Can you work these out from the drawing? Everything is in mm from the part's minimum corner. Give positions to 0.01 mm unless a question says otherwise; leave off trailing zeros. Order: outer loops, then holes, each group sorted by start corner. A loop starts at its lowest first (then second) coordinate and runs counter-clockwise, first axis right, second up. Notation, with made-up numbers: (63, -33.5) -> (87, -33.5) arc R31 ccw to (87, -5.5) -> close; hole circle Ø10 at (-26, -10.5). An arc over 180 degrees is marked (long way). One line per item, written item: value.
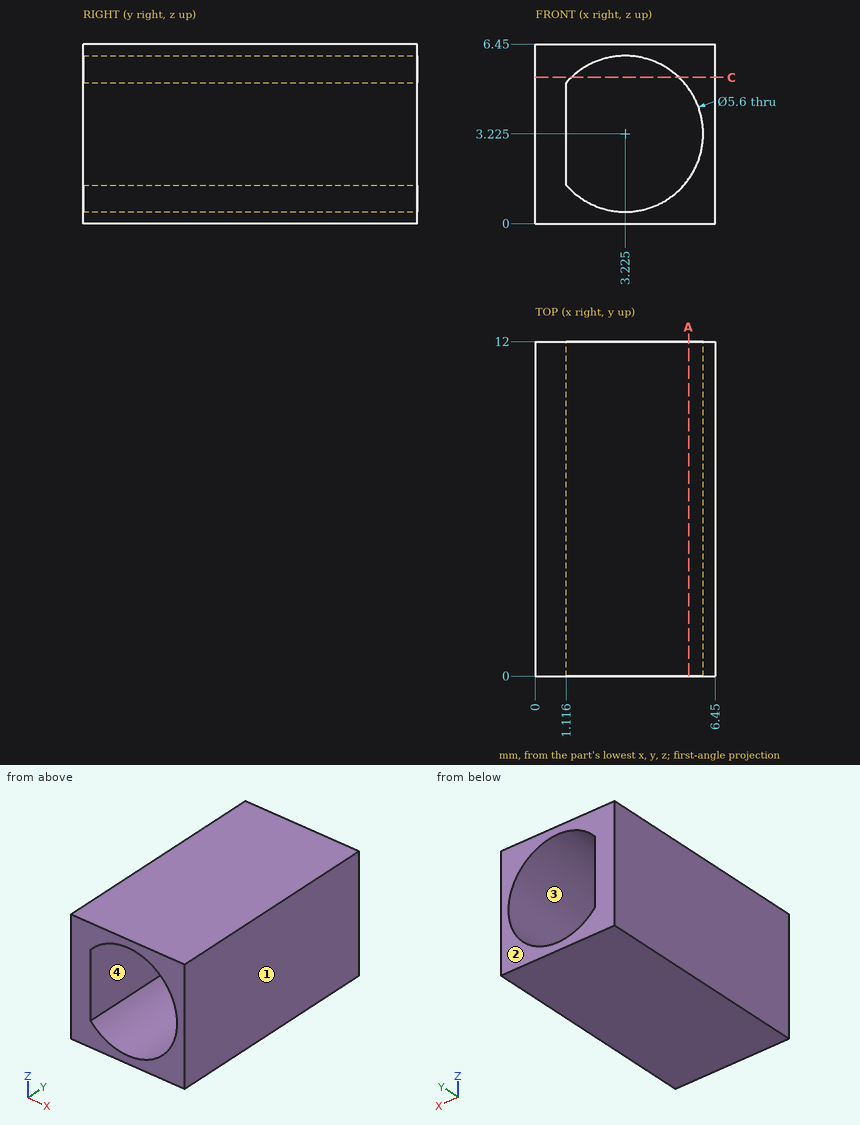
1) Suppose I cut it at A-A, the plane x = 5.5. Write out the boundary of the cut face in (y, z).
Answer below:
outline: (0, 0) -> (12, 0) -> (12, 1.59) -> (0, 1.59) -> close; (0, 4.86) -> (12, 4.86) -> (12, 6.45) -> (0, 6.45) -> close
2) Suppose I cut it at C-C, the plane z = 5.25. Write out the boundary of the cut face in (x, y), then the cut area to 3 significant figures.
Answer below:
outline: (0, 0) -> (1.29, 0) -> (1.29, 12) -> (0, 12) -> close; (5.16, 0) -> (6.45, 0) -> (6.45, 12) -> (5.16, 12) -> close
area: 31.0 mm2
3) We'd pull the mould along X, two halves only. Please class the marked faces 1, 2, 3 and 4: +X half, -X half, draft (parallel to the pull), parting line (faces both ways), or undercut.
Answer below:
face 1: +X half
face 2: draft
face 3: undercut
face 4: undercut
4) If I drill on line 1 along Z through (x, y) = (1.5, 10.75); line 2 along Z through (x, y) = (2.25, 11.75); line 3 along X through (y, z) = (10.75, 1.25), over which ranges is the centre line in solid material (lowest first)?
Answer below:
line 1: z = 0 to 1.02, 5.43 to 6.45
line 2: z = 0 to 0.6, 5.85 to 6.45
line 3: x = 0 to 1.24, 5.21 to 6.45
5) For P1, Ø3, axis at x = 2.5, y = 10.5, coming from the -Z side, with a flat end and sliding along its axis, tell me the tip position at first contact or that it passes through.
Answer below:
P1: stops at z = 0
